Here's how the part is built. I have some questions about the finished solid (model axes, mm). Face numbers are marked on the shaded views. A direction names the side the tool comes from. Round coordinates to 2 decimals unless told otherwise and drop trailing zeros. Order: outer loops, then holes, each group sorted by start corner. A loop starts at its lowest first (then second) coordinate and runs counter-clockwise, first axis right, second up.
```python
from build123d import *

# Parameters (mm, degrees)
SKETCH_1_W          = 8
SKETCH_1_H          = 8
EXTRUDE_1_DEPTH     = 1.5
SKETCH_1_10_W       = 2.5
SKETCH_1_10_H       = 14
EXTRUDE_2_DEPTH     = 8.5
SKETCH_1_11_W       = 13.2
SKETCH_1_11_H       = 2.5
EXTRUDE_3_DEPTH     = 5.5
SKETCH_1_13_R       = 3
EXTRUDE_4_DEPTH     = 3
SKETCH_1_14_W       = 8.6
SKETCH_1_14_H       = 2.5
EXTRUDE_5_DEPTH     = 1
SKETCH_1_15_R       = 2
CUT_EXTRUDE_1_DEPTH = 1.4


with BuildPart() as part:
    # Sketch 1 → Extrude 1 (new body)
    with BuildSketch(Plane.XY):
        with BuildLine():
            Line((-26.5, 39.5), (26.5, 39.5))
            ThreePointArc((26.5, 39.5), (28.621320344, 38.621320344), (29.5, 36.5))
            Line((29.5, 36.5), (29.5, -36.5))
            ThreePointArc((29.5, -36.5), (28.621320344, -38.621320344), (26.5, -39.5))
            Line((26.5, -39.5), (-26.5, -39.5))
            ThreePointArc((-26.5, -39.5), (-28.621320344, -38.621320344), (-29.5, -36.5))
            Line((-29.5, -36.5), (-29.5, 36.5))
            ThreePointArc((-29.5, 36.5), (-28.621320344, 38.621320344), (-26.5, 39.5))
        make_face()
        with Locations((11.4, 8.5)):
            Rectangle(SKETCH_1_W, SKETCH_1_H, mode=Mode.SUBTRACT)
        with Locations((2.5, 17.4)):
            Rectangle(SKETCH_1_W, SKETCH_1_H, mode=Mode.SUBTRACT)
        with Locations((-6.4, 8.5)):
            Rectangle(SKETCH_1_W, SKETCH_1_H, mode=Mode.SUBTRACT)
        with Locations((2.5, -0.4)):
            Rectangle(SKETCH_1_W, SKETCH_1_H, mode=Mode.SUBTRACT)
        with Locations((-6.9, -10.56)):
            Rectangle(SKETCH_1_W, SKETCH_1_H, mode=Mode.SUBTRACT)
        with Locations((11.9, -10.56)):
            Rectangle(SKETCH_1_W, SKETCH_1_H, mode=Mode.SUBTRACT)
    extrude(amount=EXTRUDE_1_DEPTH)

    # Sketch 1_10 → Extrude 2 (add)
    with BuildSketch(Plane.XY):
        with Locations((-28.25, 14)):
            Rectangle(SKETCH_1_10_W, SKETCH_1_10_H)
        with Locations((-28.25, -5)):
            Rectangle(SKETCH_1_10_W, SKETCH_1_10_H)
    extrude(amount=-EXTRUDE_2_DEPTH)

    # Sketch 1_11 → Extrude 3 (add)
    with BuildSketch(Plane.XY):
        with Locations((12.5, 38.25)):
            Rectangle(SKETCH_1_11_W, SKETCH_1_11_H)
        with Locations((-7.9, 38.25)):
            Rectangle(SKETCH_1_11_W, SKETCH_1_11_H)
        Polygon((-21.7, -37), (-21.7, -39.5), (-8.7, -39.5), (-8.7, -37), (-21, -37), align=None)
    extrude(amount=-EXTRUDE_3_DEPTH)

    # Sketch 1_13 → Extrude 4 (add)
    with BuildSketch(Plane.XY):
        with Locations((24, 34)):
            Circle(SKETCH_1_13_R)
        with Locations((-24, 34)):
            Circle(SKETCH_1_13_R)
        with Locations((-24, -34)):
            Circle(SKETCH_1_13_R)
        with Locations((24, -34)):
            Circle(SKETCH_1_13_R)
    extrude(amount=-EXTRUDE_4_DEPTH)

    # Sketch 1_14 → Extrude 5 (add)
    with BuildSketch(Plane.XY):
        with Locations((-4.4, -38.25)):
            Rectangle(SKETCH_1_14_W, SKETCH_1_14_H)
    extrude(amount=-EXTRUDE_5_DEPTH)

    # Sketch 1_15 → Cut-Extrude 1 (cut)
    with BuildSketch(Plane.XY):
        with Locations((2.5, 9.8)):
            Circle(SKETCH_1_15_R)
        with Locations((-8.93, -4.21)):
            Circle(SKETCH_1_15_R)
        with Locations((13.93, -4.21)):
            Circle(SKETCH_1_15_R)
        with Locations((2.5, -6.444870341)):
            Circle(SKETCH_1_15_R)
    extrude(amount=CUT_EXTRUDE_1_DEPTH, mode=Mode.SUBTRACT)


solid = part.part
```
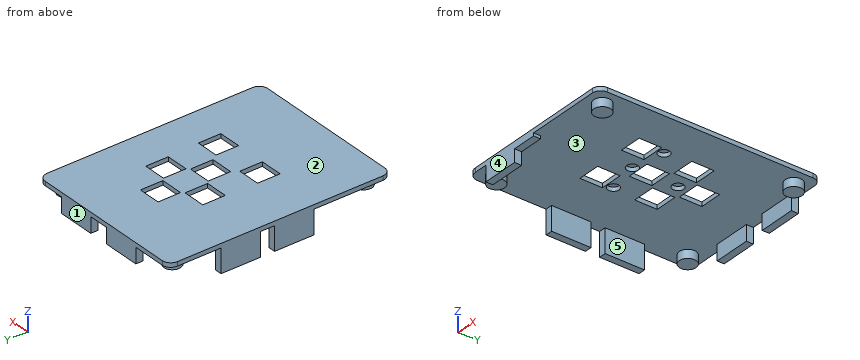
1. If we section it at A-A, the plane y = 9.8: Write out the boundary of the cut face in (x, z), and give its area (4 significant figures).
Evaluation:
outline: (-29.5, -8.5) - (-27, -8.5) - (-27, 0) - (-10.4, 0) - (-10.4, 1.5) - (-29.5, 1.5) - close; (-2.4, 0) - (0.5, 0) - (0.5, 1.4) - (4.5, 1.4) - (4.5, 0) - (7.4, 0) - (7.4, 1.5) - (-2.4, 1.5) - close; (15.4, 0) - (29.5, 0) - (29.5, 1.5) - (15.4, 1.5) - close
area: 80.15 mm2
2. If we section it at B-B, the plane x = 13.93: Write out the boundary of the cut face in (y, z), and give its area (3 significant figures).
Evaluation:
outline: (-39.5, 0) - (-14.56, 0) - (-14.56, 1.5) - (-39.5, 1.5) - close; (-6.56, 0) - (-6.21, 0) - (-6.21, 1.4) - (-2.21, 1.4) - (-2.21, 0) - (4.5, 0) - (4.5, 1.5) - (-6.56, 1.5) - close; (12.5, 0) - (37, 0) - (37, -5.5) - (39.5, -5.5) - (39.5, 1.5) - (12.5, 1.5) - close
area: 103 mm2
3. I need wall thicknesses on probe 1 along Y at (x, z) = (13.93, 0.7); probe 2 along X at (y, z) = (-13, 0.25); probe 3 along Z at (x, y) = (1, 22.5). Which ranges of each line are inside material? Lowest first, please.
Evaluation:
probe 1: y = -39.5 to -14.56, -6.56 to -6.21, -2.21 to 4.5, 12.5 to 39.5
probe 2: x = -29.5 to -10.9, -2.9 to 7.9, 15.9 to 29.5
probe 3: z = 0 to 1.5
4. If we section it at C-C, the plane x = 2.5: Write out the boundary of the cut face in (y, z), and give its area (3 significant figures).
Evaluation:
outline: (-39.5, 0) - (-8.44, 0) - (-8.44, 1.4) - (-4.44, 1.4) - (-4.44, 0) - (-4.4, 0) - (-4.4, 1.5) - (-39.5, 1.5) - close; (3.6, 0) - (7.8, 0) - (7.8, 1.4) - (11.8, 1.4) - (11.8, 0) - (13.4, 0) - (13.4, 1.5) - (3.6, 1.5) - close; (21.4, 0) - (39.5, 0) - (39.5, 1.5) - (21.4, 1.5) - close
area: 83.3 mm2
5. If we section it at D-D, the plane y = -34: Write out the boundary of the cut face in (x, z), and give its area (4 significant figures).
Evaluation:
outline: (-29.5, 0) - (-27, 0) - (-27, -3) - (-21, -3) - (-21, 0) - (21, 0) - (21, -3) - (27, -3) - (27, 0) - (29.5, 0) - (29.5, 1.5) - (-29.5, 1.5) - close
area: 124.5 mm2
6. If we mould it in two halves opening along Y, with no side actions, what happens to the marked faces 1, 2 and 3? For each: released by +Y, released by -Y, zero draft, split by the parting line, or undercut.
Evaluation:
face 1: released by +Y
face 2: zero draft
face 3: undercut
7. I'm going to push flat-ended pins straight in: P1, Ø2, axis at x = 2, y = -5.5, coming from the -Z side; P2, Ø2, axis at x = -29, z = -6, coming from the +Y side; P3, Ø5, axis at y = -30.5, z = -4.5, coming from the -X side. Where does each tip first touch, or does it pass through?
Evaluation:
P1: stops at z = 0
P2: stops at y = 21
P3: stops at x = -26.6
8. On a 3-axis mill with a long thin cutter (end or side, diameter ignored), from which of +Z, -Z, +X, -X, +Y, -Y can I reach the whole of each face in a straight line? I mean the marked faces 4 and 5. Say none if no direction works.
Evaluation:
face 4: +Z, -Z, +X, -X, -Y
face 5: -Z, +X
